Read the model definition and answer for the solid it produces. Units are mm, in the model's axes. Round coordinates to 2 decimals unless told otherwise and drop trailing zeros. Order: outer loops, then holes, each group sorted by start corner. A loop starts at its lowest first (then second) coordinate and runs counter-clockwise, first axis right, second up. Notation, with made-up numbers: M 13,-6 L 17,-6 A25 ccw 17,20 Z; hole C -7,33 d11. An arc over 180 degrees is marked long. Answer as CSV lines item,"result".
```python
from build123d import *

# Parameters (mm, degrees)
SKETCH1_R           = 3.3
BOSS_EXTRUDE1_DEPTH = 2.5


with BuildPart() as part:
    # Sketch1 → Boss-Extrude1 (new, symmetric)
    with BuildSketch(Plane(origin=(0, 0, 0), x_dir=(1, 0, 0), z_dir=(0, 1, 0))):
        Polygon((8.051309858, -0.713962815), (4.643964864, 6.615657463), (-3.407344994, 7.329620279), (-8.051309858, 0.713962815), (-4.643964864, -6.615657463), (3.407344994, -7.329620279), align=None)
        with Locations(Location((0, 0, 0), (0, 0, 270))):
            Circle(SKETCH1_R, mode=Mode.SUBTRACT)
    extrude(amount=BOSS_EXTRUDE1_DEPTH, both=True)

    # Sketch2 → Cut-Revolve1 (revolve, cut)
    with BuildSketch(Plane.XY, mode=Mode.PRIVATE) as cut_revolve1_sk:
        Polygon((6.3, 3), (8.3, 3), (8.3, 1.5), align=None)
    cut_revolve1 = revolve(cut_revolve1_sk.sketch.rotate(Axis((0, 3.572353643, 0), (0, -1, 0)), 245.067539953), axis=Axis((0, 3.572353643, 0), (0, -1, 0)), mode=Mode.SUBTRACT)

    # Mirror1: Cut-Revolve1 across plane
    add(cut_revolve1.mirror(Plane.ZX), mode=Mode.SUBTRACT)


solid = part.part
```
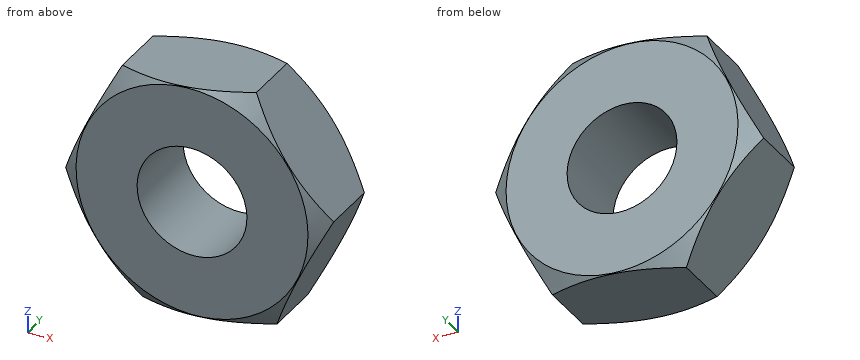
Item 1: Flat-ended cylindrical pins translate along their axes: pin 1 (2 mm diameter, centred on x = 5, y = 1.5, fed in from +Z); pin 2 (4 mm diameter, centred on x = 0, z = 0, fed in from -Y); pin 3 (3 mm diameter, centred on x = 1, y = 1, fed in from +Z); pin 4 (3 mm diameter, centred on x = 6, y = 0, fed in from -Z). Find the tip coordinate at first contact, or state that the pin passes through.
Ans:
pin 1,"z = 6.49"
pin 2,"through"
pin 3,"z = 7.25"
pin 4,"z = -6.63"
Item 2: A cutting plane is placed at C-C, the plane y = 2.15. Determine the outline of the cut face in (x, z), and give its area (3 significant figures).
Ans:
outline,"M -7.4,0.68 A7.43 ccw -7.17,-1.97 L -4.29,-6.07 A7.43 ccw -1.87,-7.19 L 3.11,-6.75 A7.43 ccw 5.29,-5.22 L 7.4,-0.68 A7.43 ccw 7.17,1.97 L 4.29,6.07 A7.43 ccw 1.87,7.19 L -3.11,6.75 A7.43 ccw -5.29,5.22 Z; hole C 0,0 d6.6"
area,"131 mm2"
Item 3: A cutting plane is placed at A-A, the plane y = 0.6. Determine the outline of the cut face in (x, z), and give its area (3 significant figures).
Ans:
outline,"M -8.05,-0.71 L -3.41,-7.33 L 4.64,-6.62 L 8.05,0.71 L 3.41,7.33 L -4.64,6.62 Z; hole C 0,0 d6.6"
area,"136 mm2"
Item 4: Find the intervals of material crossed by probe 1 along X at (y, z) = (-1.5, -0.5); probe 2 along X at (y, z) = (-0.85, 0); probe 3 along Z at (x, y) = (-2.5, 0.1), in increasing order. Write a range as [from, to].
Ans:
probe 1,"[-7.95, -3.26], [3.26, 7.49]"
probe 2,"[-7.72, -3.3], [3.3, 7.72]"
probe 3,"[-7.25, -2.15], [2.15, 6.81]"
Item 5: A cutting plane is placed at B-B, the plane z = 0. Determine the outline of the cut face in (x, y).
Ans:
outline,"M -7.72,-1.94 L -6.97,-2.5 L -3.3,-2.5 L -3.3,2.5 L -6.97,2.5 L -7.72,1.94 Z; M 3.3,-2.5 L 6.97,-2.5 L 7.72,-1.94 L 7.72,1.94 L 6.97,2.5 L 3.3,2.5 Z"
